Geometry: see drawing. Coordinates: mm, zero at the bounding-box minimum. A direction names the side the tool comes from. Give positions to 0.01 mm unless a question says otherwise; leave off trailing zeros. Order: outer loops, then holes, each group sorted by start corner. A loop starts at its lowest first (then second) coordinate and runs counter-clockwise, first axis right, second up. Notation, with made-up numbers: (36.25, 19) - (59.25, 19) arc R13 ccw to (59.25, 42) - close; hole circle Ø3 at (26, -27). An arc over 180 degrees is marked (long way). One line per question, with ' | ' between items. Start each with the question number.
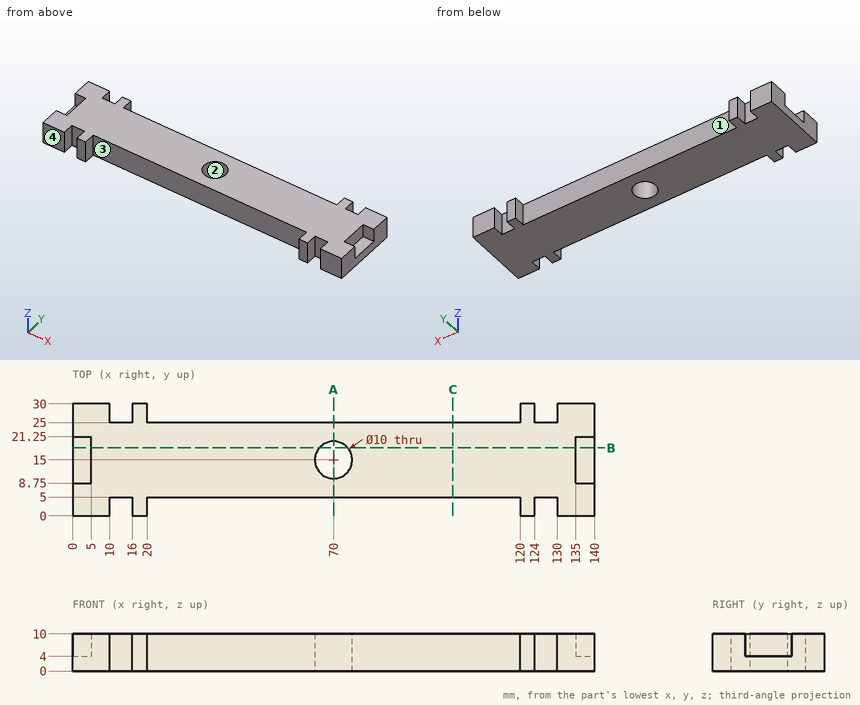
(1) Cut plane C-C, the plane x = 102. Return the cut outline in (y, z).
(2) Cut plane B-B, the plane y = 18.25. Return the cut outline in (x, z).
(3) Contact query for flat-ended pins moving along their axis: P1, Ø1.5, axis at y = 27.5, z = 3, coming from the -X side; P2, Ø3, axis at y = 12, z = 6, coming from the -X side; P3, Ø5, axis at x = 13, z = 7, coming from the +Y side; P4, Ø1.5, axis at x = 125, z = 5.5, coming from the -Y side. Output: stop coordinate, or through.
(4) Access query for the marked faces 1 and 2. Directions: +Z, -Z, +X, -X, +Y, -Y. A direction counts if a zero-diameter tool reaches every point of the face in a straight line with its end or side. Return the directions, or none.
(5) Material intervals for line 1 along X through (y, z) = (3, 6); line 2 along X through (y, z) = (14.75, 7); line 3 along Y through (x, z) = (70, 3), sorted ascending. Write a range as from..to.
(6) Pull-direction query (X, two-part tool) for the marked faces 3 and 4; classes: +X half, -X half, draft (parallel to the pull), parting line (faces both ways), or undercut.
(7) Cut plane A-A, the plane x = 70. Return the cut outline in (y, z).
Results are:
1) outline: (5, 0) - (25, 0) - (25, 10) - (5, 10) - close
2) outline: (0, 0) - (66.2, 0) - (66.2, 10) - (5, 10) - (5, 4) - (0, 4) - close; (73.8, 0) - (140, 0) - (140, 4) - (135, 4) - (135, 10) - (73.8, 10) - close
3) P1: x = 0 | P2: x = 5 | P3: y = 25 | P4: y = 5
4) face 1: +Z, -Z, +Y | face 2: +Z, -Z
5) line 1: 0..10, 16..20, 120..124, 130..140 | line 2: 5..65.01, 74.99..135 | line 3: 5..10, 20..25
6) face 3: undercut | face 4: draft
7) outline: (5, 0) - (10, 0) - (10, 10) - (5, 10) - close; (20, 0) - (25, 0) - (25, 10) - (20, 10) - close
